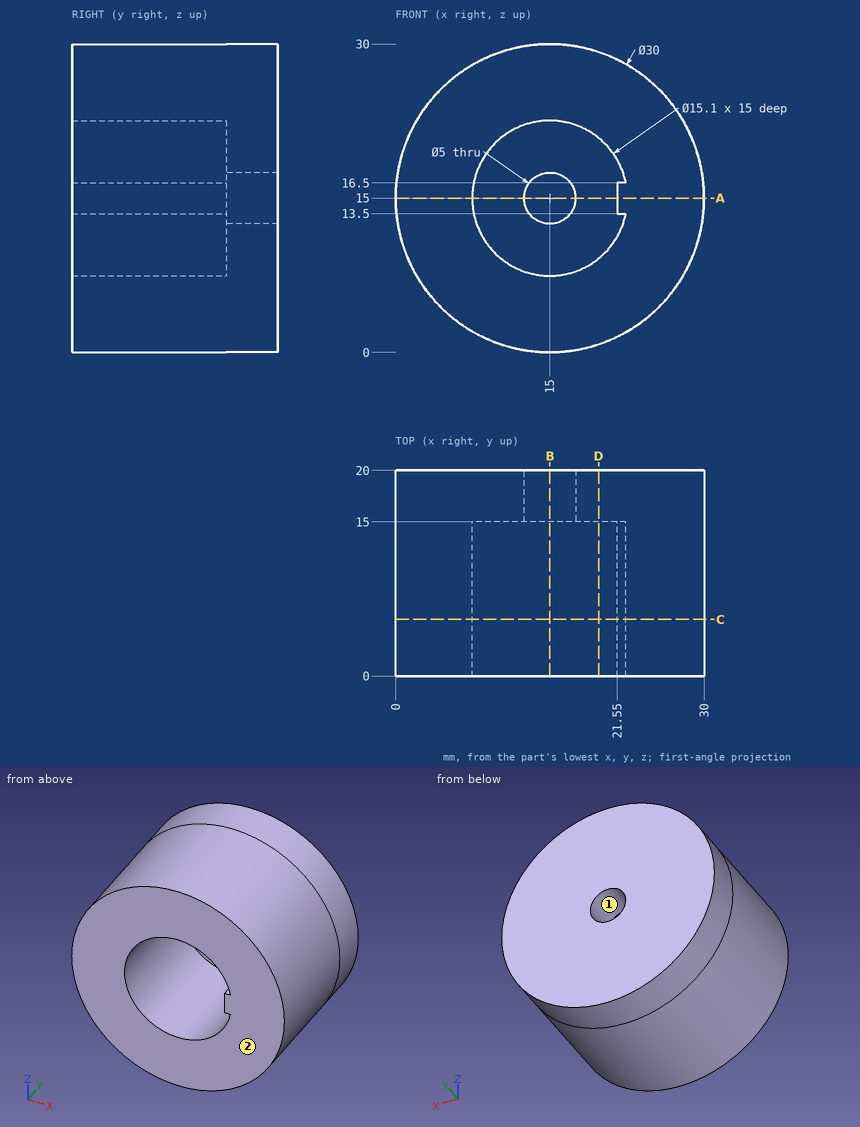
Print and shaded views of the part. All mm, measured from the part's lowest x, y and z. Round coordinates to 2 decimals unless told otherwise and drop trailing zeros. Write each loop counter-clockwise with the first axis right and the second up, starting at its lowest first coordinate (ties: lowest second). Pieces come first, ordered by that corner, then holes. Notation, with made-up numbers: (73.5, 52.25) - (122.5, 52.25) arc R22 cw to (122.5, 79.25) - close; hole circle Ø5 at (13, -20). An arc over 180 degrees is marked (long way). One line per item, written item: value.
(1) Cut at D-D, the plane x = 19.75. Give the cut face in (y, z).
Values follow:
outline: (0, 0.77) - (20, 0.77) - (20, 29.23) - (0, 29.23) - (0, 20.87) - (15, 20.87) - (15, 9.13) - (0, 9.13) - close
(2) Two-plate mould, pull along X, no slides. Class the marked faces 1 and 2: pulls with the +X half, pulls with the -X half, needs draft (parallel to the pull), parting line crosses it, or undercut.
Values follow:
face 1: undercut
face 2: needs draft
(3) Cut at C-C, the plane y = 5.5. Give the cut face in (x, z), plus the area to 3 significant figures.
Values follow:
outline: circle Ø30 at (15, 15); hole (21.55, 13.5) - (21.55, 16.5) - (22.4, 16.5) arc R7.55 ccw (long way) to (22.4, 13.5) - close
area: 531 mm²
(4) Drop flat-ended pins along their axis: P1, Ø1.5, axis at y = 10.5, z = 21, coming from the -X side; P2, Ø0.7, axis at x = 22, y = 8, coming from the -Z side; P3, Ø2, axis at y = 7.5, z = 18.5, coming from the -X side; P4, Ø3, axis at x = 15, z = 15, coming from the +Y side. Give the stop position or say it passes through.
Values follow:
P1: stops at x = 0.95
P2: stops at z = 1.55
P3: stops at x = 0.21
P4: passes through
(5) Cut at A-A, the plane z = 15. Give the cut face in (x, y), plus the area to 4 significant figures.
Values follow:
outline: (0, 0) - (7.45, 0) - (7.45, 15) - (12.5, 15) - (12.5, 20) - (0, 20) - close; (17.5, 15) - (21.55, 15) - (21.55, 0) - (30, 0) - (30, 20) - (17.5, 20) - close
area: 363.5 mm²
(6) Cut at B-B, the plane x = 15. Give the cut face in (y, z), plus the area to 4 significant figures.
Values follow:
outline: (0, 0) - (20, 0) - (20, 12.5) - (15, 12.5) - (15, 7.45) - (0, 7.45) - close; (0, 22.55) - (15, 22.55) - (15, 17.5) - (20, 17.5) - (20, 30) - (0, 30) - close
area: 348.5 mm²
(7) Wall check: probe 1 along X at (y, z) = (11.75, 15); probe 2 along Z at (x, y) = (15, 8); probe 3 along Z at (x, y) = (15, 18.75). Give the ranges that are in metal, low to high.
Values follow:
probe 1: x = 0 to 7.45, 21.55 to 30
probe 2: z = 0 to 7.45, 22.55 to 30
probe 3: z = 0 to 12.5, 17.5 to 30
